Check sheet for the modelled part. Datum: model origin and axes. Units: mm. Face numbers are marked on the shaded views. A direction names the side the tool comes from. Round coordinates to 2 decimals unless told otherwise and drop trailing zeros. Write each loop counter-clockwise with the first axis right and the second up, starting at its lowest first coordinate (ties: lowest second). Pieces come first, ordered by that corner, then holes.
Item 1: Section check A-A, the plane x = 1.5. Record the cut outline in (y, z).
Item 2: Release check for a two-part mould opening along Y. For the marked faces 4, 5 and 6 record: pulls with the +Y half, pulls with the -Y half, needs draft (parallel to the pull), parting line crosses it, or undercut.
Item 3: Material ranges on line 1 along X through (y, z) = (6.5, 9.5); line 2 along Y through (x, z) = (-3.5, 12); line 3 along X through (y, z) = (-19, 10.25), recorded low to high.
Item 4: Depth check by flat-ended pin: pin 1 (2 mm diameter, centred on x = -1, y = -19.5, fed in from -Z); pin 2 (1.3 mm diameter, centred on y = -18, z = 12, fed in from -X); pin 3 (3.5 mm diameter, centred on x = -2, y = 4, fed in from -Z). Enter the tip coordinate at first touch or a pass-through.
Item 5: Set-up check for the marked faces 1, 2 and 3: record each of +Z, -Z, +X, -X, +Y, -Y from which the full face is reachable in a straight line by a thin tool's end or side.
Item 6: Section check D-D, the plane z = 6.25. Record the cut outline in (x, y).
Item 7: Section check B-B, the plane z = 3.25. Record the cut outline in (x, y), plus the area to 3 significant figures.
Item 8: Section check C-C, the plane y = 0. Record the cut outline in (x, z), plus the area to 3 significant figures.
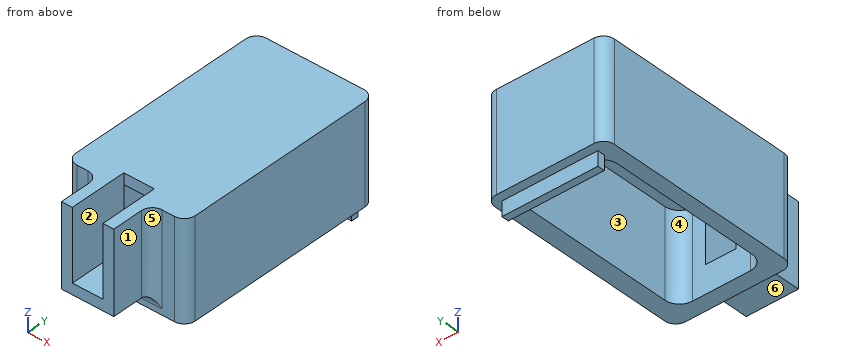
from build123d import *

# Parameters (mm, degrees)
BOSS_EXTRUDE1_DEPTH   = 14
BOSS_EXTRUDE1_2_DEPTH = 14
BOSS_EXTRUDE2_START   = 2
SKETCH1_3_W           = 1.2
SKETCH1_3_H           = 25
BOSS_EXTRUDE2_DEPTH   = 12
SKETCH2_W             = 14.2
SKETCH2_H             = 27
SKETCH2_W_2           = 12
SKETCH2_H_2           = 25
BOSS_EXTRUDE3_DEPTH   = 1.5
SKETCH3_W             = 4.2
SKETCH3_H             = 8.2
SKETCH3_H_2           = 1.5
CUT_EXTRUDE1_DEPTH    = 1
BOSS_EXTRUDE4_DEPTH   = 7
FILLET2_R             = 2
SKETCH5_W             = 13.2
SKETCH5_H             = 1
CUT_EXTRUDE2_DEPTH    = 2
FILLET4_R             = 1
BOSS_EXTRUDE7_START   = -13.5
BOSS_EXTRUDE7_DEPTH   = 13.5
BOSS_EXTRUDE8_DEPTH   = 2.3
FILLET5_R             = 1.5
SKETCH10_W            = 0.4
SKETCH10_H            = 29.4
CUT_EXTRUDE3_DEPTH    = 13.5
FILLET6_R             = 1.5


with BuildPart() as part:
    # Sketch1 → Boss-Extrude1 (new body)
    with BuildSketch(Plane.XY):
        Polygon((7.2, 13.5), (-6, 13.5), (-6, 12.5), (6, 12.5), (7.2, 12.5), align=None)
    extrude(amount=BOSS_EXTRUDE1_DEPTH)



with BuildPart() as body_2:
    # Sketch1 → Boss-Extrude1 2 (new body)
    with BuildSketch(Plane.XY):
        Polygon((6, -12.5), (-6, -12.5), (-6, -13.5), (7.2, -13.5), (7.2, -12.5), align=None)
    extrude(amount=BOSS_EXTRUDE1_2_DEPTH)


with BuildPart() as part_1:
    add(part.part)

    add(body_2.part)  # Boss-Extrude2 merges body 2
    # Sketch1<3> → Boss-Extrude2 (add)
    with BuildSketch(Plane.XY.offset(BOSS_EXTRUDE2_START)):
        Polygon((-6, 12.5), (-6, 13.5), (-7, 13.5), (-7, -13.5), (-6, -13.5), (-6, -12.5), align=None)
        with Locations((6.6, 0)):
            Rectangle(SKETCH1_3_W, SKETCH1_3_H)
    extrude(amount=BOSS_EXTRUDE2_DEPTH)

    # Sketch2 → Boss-Extrude3 (add)
    # profile 1 of 2: a face of its own
    with BuildSketch(Plane.XY.offset(14)):
        with Locations((0.1, 0)):
            Rectangle(SKETCH2_W, SKETCH2_H)
        Rectangle(SKETCH2_W_2, SKETCH2_H_2, mode=Mode.SUBTRACT)
    # profile 2 of 2: a face of its own
    with BuildSketch(Plane.XY.offset(14)):
        Rectangle(SKETCH2_W_2, SKETCH2_H_2)
    extrude(amount=BOSS_EXTRUDE3_DEPTH)

    # Sketch3 → Cut-Extrude1 (cut)
    with BuildSketch(Plane.XZ.offset(13.5)):
        with Locations((0.063870968, 9.9)):
            Rectangle(SKETCH3_W, SKETCH3_H)
        with Locations((0.063870968, 14.75)):
            Rectangle(SKETCH3_W, SKETCH3_H_2)
    extrude(amount=-CUT_EXTRUDE1_DEPTH, mode=Mode.SUBTRACT)

    # Sketch4 → Boss-Extrude4 (add)
    with BuildSketch(Plane.XZ.offset(13.5)):
        Polygon((3.663870968, 15.5), (2.163870968, 15.5), (2.163870968, 5.8), (-2.036129032, 5.8), (-2.036129032, 15.5), (-3.536129032, 15.5), (-3.536129032, 4.3), (3.663870968, 4.3), align=None)
    extrude(amount=BOSS_EXTRUDE4_DEPTH)

    # Fillet2
    fillet2_edges = [part_1.edges().sort_by_distance(p)[0] for p in [
        (-6, -12.5, 8),
        (6, -12.5, 8),
        (6, 12.5, 8),
        (-6, 12.5, 8),
    ]]
    fillet(fillet2_edges, radius=FILLET2_R)

    # Sketch5 → Cut-Extrude2 (cut)
    with BuildSketch(Plane(origin=(0, 0, 2), x_dir=(-1, 0, 0), z_dir=(0, 0, -1))):
        with Locations((-0.6, -13)):
            Rectangle(SKETCH5_W, SKETCH5_H)
    extrude(amount=CUT_EXTRUDE2_DEPTH, mode=Mode.SUBTRACT)

    # Fillet4
    fillet4_edges = [part_1.edges().sort_by_distance(p)[0] for p in [
        (3.663870968, -13.5, 9.9),
        (0.063870968, -13.5, 4.3),
        (-3.536129032, -13.5, 9.9),
    ]]
    fillet(fillet4_edges, radius=FILLET4_R)

    # Sketch8 → Boss-Extrude7 (add)
    with BuildSketch(Plane.XY.offset(15.5).offset(BOSS_EXTRUDE7_START)):
        with BuildLine():
            Line((8.4, -14.7), (8.4, 14.7))
            Line((8.4, 14.7), (-8.4, 14.7))
            Line((-8.4, 14.7), (-8.4, -14.7))
            Line((-8.4, -14.7), (-3.536129032, -14.7))
            Line((-3.536129032, -14.7), (-3.536129032, -14.5))
            ThreePointArc((-3.536129032, -14.5), (-3.829022251, -13.792893219), (-4.536129032, -13.5))
            Line((-4.536129032, -13.5), (-7, -13.5))
            Line((-7, -13.5), (-7, 13.5))
            Line((-7, 13.5), (7.2, 13.5))
            Line((7.2, 13.5), (7.2, -13.5))
            Line((7.2, -13.5), (4.663870968, -13.5))
            ThreePointArc((4.663870968, -13.5), (3.956764187, -13.792893219), (3.663870968, -14.5))
            Line((3.663870968, -14.5), (3.663870968, -14.7))
            Line((3.663870968, -14.7), (8.4, -14.7))
        make_face()
    extrude(amount=BOSS_EXTRUDE7_DEPTH)

    # Sketch9 → Boss-Extrude8 (add)
    with BuildSketch(Plane(origin=(0, 0, 2), x_dir=(-1, 0, 0), z_dir=(0, 0, -1))):
        Polygon((-5.007987006, -14.7), (5.670470917, -14.7), (5.670470917, -12.839003899), (-4.79710184, -12.839003899), align=None)
    extrude(amount=-BOSS_EXTRUDE8_DEPTH)

    # Fillet5
    fillet5_edges = [part_1.edges().sort_by_distance(p)[0] for p in [
        (3.663870968, -14.7, 9.9),
        (-3.536129032, -14.7, 9.9),
        (0.063870968, -14.7, 4.3),
    ]]
    fillet(fillet5_edges, radius=FILLET5_R)

    # Sketch10 → Cut-Extrude3 (cut)
    with BuildSketch(Plane(origin=(0, 0, 2), x_dir=(-1, 0, 0), z_dir=(0, 0, -1))):
        with Locations((8.2, 0)):
            Rectangle(SKETCH10_W, SKETCH10_H)
    extrude(amount=-CUT_EXTRUDE3_DEPTH, mode=Mode.SUBTRACT)

    # Fillet6
    fillet6_edges = [part_1.edges().sort_by_distance(p)[0] for p in [
        (8.4, 14.7, 8.75),
        (8.4, -14.7, 8.75),
        (-8, 14.7, 8.75),
        (-8, -14.7, 8.75),
    ]]
    fillet(fillet6_edges, radius=FILLET6_R)


solid = part_1.part
Values found:
1. outline: (-20.5, 4.3) - (-16.2, 4.3) arc R1.5 cw to (-14.7, 2.8) - (-14.7, 2) - (-12.5, 2) - (-12.5, 5.8) - (-20.5, 5.8) - close; (-12.5, 14) - (12.5, 14) - (12.5, 0) - (13.5, 0) - (13.5, 2) - (14.7, 2) - (14.7, 15.5) - (-12.5, 15.5) - close
2. face 4: undercut
2. face 5: pulls with the -Y half
2. face 6: needs draft
3. line 1: x = -8 to -6, 6 to 8.4
3. line 2: y = -20.5 to -12.5, 12.5 to 14.7
3. line 3: x = -3.54 to -2.04, 2.16 to 3.66
4. pin 1: stops at z = 4.3
4. pin 2: stops at x = -3.54
4. pin 3: stops at z = 14
5. face 1: +Z, -Z, +X, -Y
5. face 2: +Z, -Y
5. face 3: -Z
6. outline: (-8, -13.2) arc R1.5 ccw to (-6.5, -14.7) - (-5.04, -14.7) arc R1.5 cw to (-3.54, -16.2) - (-3.54, -20.5) - (-2.04, -20.5) - (-2.04, -12.5) - (-4, -12.5) arc R2 cw to (-6, -10.5) - (-6, 10.5) arc R2 cw to (-4, 12.5) - (4, 12.5) arc R2 cw to (6, 10.5) - (6, -10.5) arc R2 cw to (4, -12.5) - (2.16, -12.5) - (2.16, -20.5) - (3.66, -20.5) - (3.66, -16.2) arc R1.5 cw to (5.16, -14.7) - (6.9, -14.7) arc R1.5 ccw to (8.4, -13.2) - (8.4, 13.2) arc R1.5 ccw to (6.9, 14.7) - (-6.5, 14.7) arc R1.5 ccw to (-8, 13.2) - close
7. outline: (-8, -13.2) arc R1.5 ccw to (-6.5, -14.7) - (-5.04, -14.7) arc R1.5 cw to (-4.59, -14.77) - (4.71, -14.77) arc R1.5 cw to (5.16, -14.7) - (6.9, -14.7) arc R1.5 ccw to (8.4, -13.2) - (8.4, 13.2) arc R1.5 ccw to (6.9, 14.7) - (-6.5, 14.7) arc R1.5 ccw to (-8, 13.2) - close; hole (-6, -10.5) arc R2 ccw to (-4, -12.5) - (4, -12.5) arc R2 ccw to (6, -10.5) - (6, 10.5) arc R2 ccw to (4, 12.5) - (-4, 12.5) arc R2 ccw to (-6, 10.5) - close
7. area: 184 mm2
8. outline: (-8, 2) - (-6, 2) - (-6, 14) - (6, 14) - (6, 2) - (8.4, 2) - (8.4, 15.5) - (-8, 15.5) - close
8. area: 77.4 mm2
